Could you check a few things on this model? Use its own coordinates, in mm. A direction names the side the tool comes from. Round coordinates to 2 decimals unless told otherwise and drop trailing zeros. Write each loop counter-clockwise with the first axis right and the second up, starting at its lowest first coordinate (ties: lowest second). Pieces come first, ordered by that corner, then holes.
```python
from build123d import *

# Parameters (mm, degrees)
F0_W     = 101.6
F0_H     = 127
F0_R     = 6.35
F1_DEPTH = 9.525
F4_DEPTH = 1000.125
F6_DEPTH = 581.025
F7_W     = 361.95
F7_H     = 82.55
F7_R     = 4.7625
F8_DEPTH = 9.525


# Not quite as in the source:
# - a length typed as a fraction of an inch, garbled in the dataset ("3 / 203.2 mm" for 3/8 in), is restored


with BuildPart() as f1:
    # F0 (on Top) → F1 (new body)
    with BuildSketch(Plane.XY):
        with Locations((50.8, 63.5)):
            Rectangle(F0_W, F0_H)
        with Locations((19.05, 19.05)):
            Circle(F0_R, mode=Mode.SUBTRACT)
        with Locations((82.55, 19.05)):
            Circle(F0_R, mode=Mode.SUBTRACT)
        with Locations((19.05, 107.95)):
            Circle(F0_R, mode=Mode.SUBTRACT)
        with Locations((82.55, 107.95)):
            Circle(F0_R, mode=Mode.SUBTRACT)
    extrude(amount=F1_DEPTH)

    # F3 (on offset) → F4 (join)
    with BuildSketch(Plane.XY.offset(9.525)):
        with BuildLine():
            Line((31.75, 38.1), (69.85, 38.1))
            ThreePointArc((69.85, 38.1), (74.3401280605, 39.9598719395), (76.2, 44.45))
            Line((76.2, 44.45), (76.2, 82.55))
            ThreePointArc((76.2, 82.55), (74.3401280605, 87.0401280605), (69.85, 88.9))
            Line((69.85, 88.9), (31.75, 88.9))
            ThreePointArc((31.75, 88.9), (27.2598719395, 87.0401280605), (25.4, 82.55))
            Line((25.4, 82.55), (25.4, 44.45))
            ThreePointArc((25.4, 44.45), (27.2598719395, 39.9598719395), (31.75, 38.1))
        make_face()
        with BuildLine():
            ThreePointArc((71.4375, 49.2125), (69.5776280605, 44.7223719395), (65.0875, 42.8625))
            Line((65.0875, 42.8625), (36.5125, 42.8625))
            ThreePointArc((36.5125, 42.8625), (32.0223719395, 44.7223719395), (30.1625, 49.2125))
            Line((30.1625, 49.2125), (30.1625, 77.7875))
            ThreePointArc((30.1625, 77.7875), (32.0223719395, 82.2776280605), (36.5125, 84.1375))
            Line((36.5125, 84.1375), (65.0875, 84.1375))
            ThreePointArc((65.0875, 84.1375), (69.5776280605, 82.2776280605), (71.4375, 77.7875))
            Line((71.4375, 77.7875), (71.4375, 49.2125))
        make_face(mode=Mode.SUBTRACT)
    extrude(amount=F4_DEPTH)

    # F5 (on face) → F6 (join)
    with BuildSketch(Plane.XZ.offset(-38.1)):
        with BuildLine():
            Line((31.75, 958.85), (69.85, 958.85))
            ThreePointArc((69.85, 958.85), (74.3401280605, 960.7098719395), (76.2, 965.2))
            Line((76.2, 965.2), (76.2, 1003.3))
            ThreePointArc((76.2, 1003.3), (74.3401280605, 1007.7901280605), (69.85, 1009.65))
            Line((69.85, 1009.65), (31.75, 1009.65))
            ThreePointArc((31.75, 1009.65), (27.2598719395, 1007.7901280605), (25.4, 1003.3))
            Line((25.4, 1003.3), (25.4, 965.2))
            ThreePointArc((25.4, 965.2), (27.2598719395, 960.7098719395), (31.75, 958.85))
        make_face()
        with BuildLine():
            ThreePointArc((71.4375, 969.9625), (69.5776280605, 965.4723719395), (65.0875, 963.6125))
            Line((65.0875, 963.6125), (36.5125, 963.6125))
            ThreePointArc((36.5125, 963.6125), (32.0223719395, 965.4723719395), (30.1625, 969.9625))
            Line((30.1625, 969.9625), (30.1625, 998.5375))
            ThreePointArc((30.1625, 998.5375), (32.0223719395, 1003.0276280605), (36.5125, 1004.8875))
            Line((36.5125, 1004.8875), (65.0875, 1004.8875))
            ThreePointArc((65.0875, 1004.8875), (69.5776280605, 1003.0276280605), (71.4375, 998.5375))
            Line((71.4375, 998.5375), (71.4375, 969.9625))
        make_face(mode=Mode.SUBTRACT)
    extrude(amount=F6_DEPTH)

    # F7 (on face) → F8 (join)
    with BuildSketch(Plane.XZ.offset(542.925)):
        with Locations((50.8, 968.375)):
            Rectangle(F7_W, F7_H)
        with Locations((-111.125, 946.15)):
            Circle(F7_R, mode=Mode.SUBTRACT)
        with Locations((-66.675, 946.15)):
            Circle(F7_R, mode=Mode.SUBTRACT)
        with Locations((168.275, 946.15)):
            Circle(F7_R, mode=Mode.SUBTRACT)
        with Locations((212.725, 946.15)):
            Circle(F7_R, mode=Mode.SUBTRACT)
        with Locations((-111.125, 990.6)):
            Circle(F7_R, mode=Mode.SUBTRACT)
        with Locations((-66.675, 990.6)):
            Circle(F7_R, mode=Mode.SUBTRACT)
        with Locations((168.275, 990.6)):
            Circle(F7_R, mode=Mode.SUBTRACT)
        with Locations((212.725, 990.6)):
            Circle(F7_R, mode=Mode.SUBTRACT)
    extrude(amount=F8_DEPTH)


solid = f1.part
```
Q1. I'm going to push flat-ended pins straight in: pin 1 Ø23 at (x, y) = (50, -377) entering from -Z; pin 2 Ø7.5 at (x, z) = (58, 5.5) entering from -Y; pin 3 Ø7.5 at (x, y) = (-9.5, -548.5) entering from -Z. Where does each tip first touch, or does it pass through?
Q2. If I drill on L1, parallel to Y at x = 19.05, z = 2; L2, parallel to X at y = -548, z = 946.15 (1 decimal); L3, parallel to Y at x = 38.5, z = 649, over which ranges is the centre line in solid material (lowest first)?
Q3. Imagine slicing it at C-C, the plane x = -45. Write out the boundary of the cut face in (y, z) (3 decimals).
Q4. Imagine slicing it at A-A, the plane y = -280. Write out the boundary of the cut face in (x, z).
Q5. We'd pull the mould along Y, two halves only. Please class faces 1 (the flat face through (30.162, 63, 503)), 2 (the flat face through (50, 64, 0)), 3 (the flat face through (48, -552.45, 969)): pulls with the +Y half, pulls with the -Y half, needs draft (parallel to the pull), parting line crosses it, or undercut.
Q6. Imagine slicing it at B-B, the plane z = 163.5. Write out the boundary of the cut face in (x, y).
Q7. On a 3-axis mill with a long thin cutter (end or side, diameter ignored), from which of +Z, -Z, +X, -X, +Y, -Y can I reach the whole of each face in a straight line? I mean faces 4 (the flat face through (50, -254, 1009.65)), 5 (the flat face through (51, -248, 963.612)), 6 (the flat face through (51, 64, 9.525)). Say none if no direction works.
Results found:
1. pin 1: stops at z = 958.85
1. pin 2: stops at y = 0
1. pin 3: stops at z = 927.1
2. L1: y = 0 to 12.7, 25.4 to 101.6, 114.3 to 127
2. L2: x = -130.2 to -115.9, -106.4 to -71.4, -61.9 to 163.5, 173 to 208, 217.5 to 231.8
2. L3: y = 38.1 to 42.86, 84.14 to 88.9
3. outline: (-552.45, 927.1) - (-542.925, 927.1) - (-542.925, 1009.65) - (-552.45, 1009.65) - close
4. outline: (25.4, 965.2) arc R6.35 ccw to (31.75, 958.85) - (69.85, 958.85) arc R6.35 ccw to (76.2, 965.2) - (76.2, 1003.3) arc R6.35 ccw to (69.85, 1009.65) - (31.75, 1009.65) arc R6.35 ccw to (25.4, 1003.3) - close; hole (30.16, 969.96) arc R6.35 ccw to (36.51, 963.61) - (65.09, 963.61) arc R6.35 ccw to (71.44, 969.96) - (71.44, 998.54) arc R6.35 ccw to (65.09, 1004.89) - (36.51, 1004.89) arc R6.35 ccw to (30.16, 998.54) - close
5. face 1: undercut
5. face 2: needs draft
5. face 3: pulls with the -Y half
6. outline: (25.4, 44.45) arc R6.35 ccw to (31.75, 38.1) - (69.85, 38.1) arc R6.35 ccw to (76.2, 44.45) - (76.2, 82.55) arc R6.35 ccw to (69.85, 88.9) - (31.75, 88.9) arc R6.35 ccw to (25.4, 82.55) - close; hole (30.16, 49.21) arc R6.35 ccw to (36.51, 42.86) - (65.09, 42.86) arc R6.35 ccw to (71.44, 49.21) - (71.44, 77.79) arc R6.35 ccw to (65.09, 84.14) - (36.51, 84.14) arc R6.35 ccw to (30.16, 77.79) - close
7. face 4: +Z, +X, -X, +Y, -Y
7. face 5: none
7. face 6: +Z
